Design review of the part built by this model. Coordinates are the model's own, in mm. A direction names the side the tool comes from. Coordinates: 2 decimals unless noted, no trailing zeros. Loops run counter-clockwise (first coordinate to the right, second up) from the corner with the lowest first, then second, coordinate; pieces in that order, holes last. Notation, with made-up numbers: (-28, -9) - (-15, -9) arc R21 ccw to (-15, -1) - close; hole circle Ø5 at (-11, 22.25). An arc over 180 degrees is marked (long way). Answer in a Markdown table with one row per item. Add a question column.
(1) Clearance check with flat-ended pins moving along their axes: pin 1 (4 mm diameter, centred on y = 21, z = 5, fed in from +X); pin 2 (1.9 mm diameter, centred on x = -5.5, z = 5, fed in from -Y); pin 3 (5.5 mm diameter, centred on x = -8.5, z = 4.5, fed in from +Y). State where each tip first meets the part, or that it passes through.
(2) The part is to be moulded in two halves that separate along Y. For faces 5 (the face through (-9, 25, 11)), 6 (the face through (4, 5.4, 5)), 7 (the face through (-12.5, 34.9, 5.4)), 8 (the face through (-5, 21, 5)), say which applies: released by +Y, released by -Y, zero draft, split by the parting line, or undercut.
(3) For faces 1 (the face through (-5, 7.3, 5.4)), 2 (the face through (7.8, 42.4, 5.4)), 3 (the face through (-2.5, 34.9, 5.4)), 4 (the face through (0.338, 2.738, 8.078)), list the 3-axis set-ups (+Z, -Z, +X, -X, +Y, -Y) from which the entire face can be reached by the end or side of a thin tool; tool diameter is ignored.
(4) We need section B-B, the plane x = -1. Write out the cut boundary in (y, z).
(5) We need section C-C, the plane y = 4. Write out the cut boundary in (x, z).
(6) We need section A-A, the plane z = 1.5. Write out the cut boundary in (x, y), plus the area to 3 significant figures.
(7) To check wall thickness, follow L1, parallel to Z at x = 0, y = 2; L2, parallel to X at y = 1.35, z = 5.5; L3, parallel to Y at x = 2.5, z = 2.75. State the ranges of each line that lie inside material, in increasing order. Write a range as [from, to].
(8) We need section D-D, the plane z = 4. Write out the cut boundary in (x, y), plus the area to 3 significant figures.
from build123d import *

# Parameters (mm, degrees)
EXTRUDE_1_DEPTH     = 11
CHAMFER_2_SIZE      = 5
CHAMFER_3_SIZE      = 1
SKETCH_2_R          = 2.6
CUT_EXTRUDE_1_DEPTH = 53.163205423
SKETCH_3_R          = 5
CUT_EXTRUDE_2_DEPTH = 5


with BuildPart() as part:
    # Эскиз1 → Бобышка-Вытянуть1 (new body)
    with BuildSketch(Plane.XY):
        Polygon((-10, 0.4), (-3.7, 0.4), (-3.7, 0), (3.7, 0), (3.7, 0.4), (10, 0.4), (10, 5.4), (-5, 5.4), (-5, 37.4), (9, 37.4), (9, 43.4), (8.6, 43.4), (7, 41.4), (-32, 41.4), (-33.6, 43.4), (-34, 43.4), (-34, 37.4), (-10, 37.4), align=None)
    extrude(amount=EXTRUDE_1_DEPTH)

    # Фаска2
    chamfer_2_edges = [part.edges().sort_by_distance(p)[0] for p in [
        (-10, 37.4, 5.5),
        (-5, 37.4, 5.5),
        (-5, 5.4, 5.5),
    ]]
    chamfer(chamfer_2_edges, length=CHAMFER_2_SIZE)

    # Фаска3
    chamfer_3_edges = [part.edges().sort_by_distance(p)[0] for p in [
        (-34, 37.4, 5.5),
        (9, 37.4, 5.5),
    ]]
    chamfer(chamfer_3_edges, length=CHAMFER_3_SIZE)

    # Эскиз2 → Вырез-Вытянуть1 (cut, through all)
    with BuildSketch(Plane(origin=(0, 5.4, 0), x_dir=(1, 0, 0), z_dir=(0, 1, 0))):
        with Locations(Location((0, -5.5, 0), (0, 0, 180))):
            Circle(SKETCH_2_R)
    extrude(amount=-CUT_EXTRUDE_1_DEPTH, mode=Mode.SUBTRACT)

    # Эскиз3 → Вырез-Вытянуть2 (cut)
    with BuildSketch(Plane(origin=(0, 5.4, 0), x_dir=(1, 0, 0), z_dir=(0, 1, 0))):
        with Locations((0, -5.5)):
            Circle(SKETCH_3_R)
    extrude(amount=CUT_EXTRUDE_2_DEPTH, mode=Mode.SUBTRACT)


solid = part.part
Responses:
| question | item | result |
|---|---|---|
| 1 | pin 1 | stops at x = -5 |
| 1 | pin 2 | stops at y = 0.4 |
| 1 | pin 3 | stops at y = 41.4 |
| 2 | face 5 | zero draft |
| 2 | face 6 | undercut |
| 2 | face 7 | released by -Y |
| 2 | face 8 | undercut |
| 3 | face 1 | +X |
| 3 | face 2 | +Z, -Z, +Y |
| 3 | face 3 | +Z, -Z, +X |
| 3 | face 4 | -Y |
| 4 | outline | (0, 0) - (6.4, 0) - (6.4, 0.6) - (5.4, 0.6) - (5.4, 3.1) - (0, 3.1) - close; (0, 7.9) - (5.4, 7.9) - (5.4, 10.4) - (6.4, 10.4) - (6.4, 11) - (0, 11) - close; (36.4, 0) - (41.4, 0) - (41.4, 11) - (36.4, 11) - close |
| 5 | outline | (-10, 0) - (10, 0) - (10, 11) - (-10, 11) - close; hole circle Ø5.2 at (0, 5.5) |
| 6 | outline | (-34, 38.4) - (-33, 37.4) - (-15, 37.4) - (-10, 32.4) - (-10, 0.4) - (-3.7, 0.4) - (-3.7, 0) - (3.7, 0) - (3.7, 0.4) - (10, 0.4) - (10, 5.4) - (-3, 5.4) - (-3, 8.4) - (-5, 10.4) - (-5, 32.4) - (0, 37.4) - (8, 37.4) - (9, 38.4) - (9, 43.4) - (8.6, 43.4) - (7, 41.4) - (-32, 41.4) - (-33.6, 43.4) - (-34, 43.4) - close |
| 6 | area | 472 mm2 |
| 7 | L1 | z = [0, 2.9], [8.1, 11] |
| 7 | L2 | x = [-10, -2.6], [2.6, 10] |
| 7 | L3 | y = [0, 5.4], [37.4, 41.4] |
| 8 | outline | (-34, 38.4) - (-33, 37.4) - (-15, 37.4) - (-10, 32.4) - (-10, 0.4) - (-3.7, 0.4) - (-3.7, 0) - (-2.12, 0) - (-2.12, 5.4) - (-4.77, 5.4) - (-4.77, 10.17) - (-5, 10.4) - (-5, 32.4) - (0, 37.4) - (8, 37.4) - (9, 38.4) - (9, 43.4) - (8.6, 43.4) - (7, 41.4) - (-32, 41.4) - (-33.6, 43.4) - (-34, 43.4) - close; (2.12, 0) - (3.7, 0) - (3.7, 0.4) - (10, 0.4) - (10, 5.4) - (2.12, 5.4) - close |
| 8 | area | 442 mm2 |
